```python
from build123d import *

# Parameters (mm, degrees)
F0_W     = 15.875
F0_H     = 31.75
F1_DEPTH = 12.7
F2_R     = 4.7625
F3_DEPTH = 12.7
F4_R     = 2.7051
F5_DEPTH = 31.75


with BuildPart() as f1:
    # F0 (on Top) → F1 (new body)
    with BuildSketch(Plane.XY):
        with Locations((7.9375, 15.875)):
            Rectangle(F0_W, F0_H)
    extrude(amount=F1_DEPTH)

    # F2 (on face) → F3 (cut, through all)
    with BuildSketch(Plane.XY.offset(12.7)):
        with Locations((7.9375, 22.225)):
            Circle(F2_R)
    extrude(amount=-F3_DEPTH, mode=Mode.SUBTRACT)

    # F4 (on face) → F5 (cut, through all)
    with BuildSketch(Plane.XZ):
        with Locations((7.9375, 6.35)):
            Circle(F4_R)
    extrude(amount=-F5_DEPTH, mode=Mode.SUBTRACT)


solid = f1.part
```
Could you check a few things on this model? Use its own coordinates, in mm. Give positions to 0.01 mm unless a question says otherwise; leave off trailing zeros. Order: outer loops, then holes, each group sorted by start corner. A loop starts at its lowest first (then second) coordinate and runs counter-clockwise, first axis right, second up.
Q1. If I drill on line 1 along X through (y, z) = (10, 6.35) (3 decimals); line 2 along X through (y, z) = (21, 5) (3 decimals); line 3 along Z through (x, y) = (8.5, 27), over which ranges is the centre line in solid material (lowest first)?
Q2. Suppose I cut it at D-D, the plane x = 8.5. Write out the boundary of the cut face in (y, z), and give its area (3 significant figures).
Q3. Suppose I cut it at C-C, the plane x = 3.75. Write out the boundary of the cut face in (y, z), and give its area (3 significant figures).
Q4. We'd pull the mould along Z, two halves only. Please class faces 1 (the cylindrical face through (10.52, 28.91, 7.16)), 2 (the flat face through (15.875, 16, 6)), 3 (the flat face through (8, 16, 0)): +Z half, -Z half, draft (parallel to the pull), parting line (faces both ways), or undercut.
Solution:
1. line 1: x = 0 to 5.232, 10.643 to 15.875
1. line 2: x = 0 to 3.335, 12.54 to 15.875
1. line 3: z = 0 to 3.7, 9 to 12.7
2. outline: (0, 0) - (17.5, 0) - (17.5, 3.7) - (0, 3.7) - close; (0, 9) - (17.5, 9) - (17.5, 12.7) - (0, 12.7) - close; (26.95, 0) - (31.75, 0) - (31.75, 3.7) - (26.95, 3.7) - close; (26.95, 9) - (31.75, 9) - (31.75, 12.7) - (26.95, 12.7) - close
2. area: 165 mm2
3. outline: (0, 0) - (19.96, 0) - (19.96, 12.7) - (0, 12.7) - close; (24.49, 0) - (31.75, 0) - (31.75, 12.7) - (24.49, 12.7) - close
3. area: 346 mm2
4. face 1: undercut
4. face 2: draft
4. face 3: -Z half
